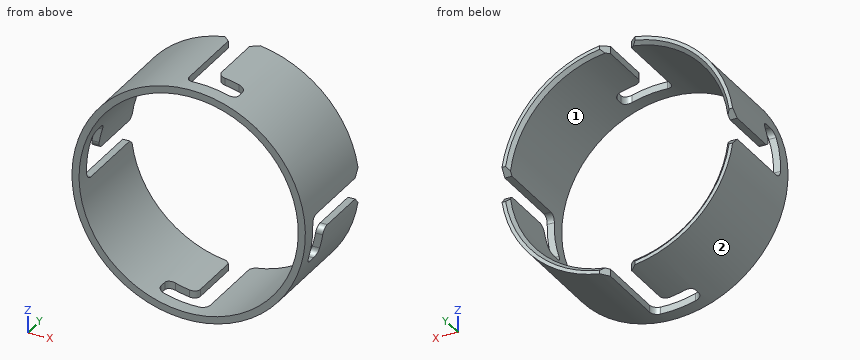
from build123d import *

# Parameters (mm, degrees)
SKETCH2_W                    = 5
SKETCH2_H                    = 72.15
CUT_EXTRUDE1_DEPTH           = 83.55
FILLET1_R                    = 5
CHAMFER1_SIZE                = 5
FILLET3_R                    = 5
CIRPATTERN1_COUNT            = 4
FILLET1_OF_CIRPATTERN1_R     = 5
CHAMFER1_OF_CIRPATTERN1_SIZE = 5
FILLET3_OF_CIRPATTERN1_R     = 5
CHAMFER2_SIZE                = 2.5


with BuildPart() as part:
    # Sketch2 → Revolve1 (revolve)
    with BuildSketch(Plane(origin=(0, 0, 0), x_dir=(0, 0, -1), z_dir=(1, 0, 0))):
        with Locations((-80.05, 36.075)):
            Rectangle(SKETCH2_W, SKETCH2_H)
    revolve(axis=Axis((0, -3.6075, 0), (0, 1, 0)))

    # Sketch3 → Cut-Extrude1 (cut, through all)
    with BuildSketch(Plane(origin=(0, 0, 0), x_dir=(0, 0, -1), z_dir=(1, 0, 0))):
        Polygon((-7.5, 72.15), (7.5, 72.15), (7.5, 10), (-27.5, 10), (-27.5, 25), (-7.5, 25), align=None)
    cut_extrude1 = extrude(amount=-CUT_EXTRUDE1_DEPTH, mode=Mode.SUBTRACT)

    # Fillet1
    fillet1_edges = [part.edges().sort_by_distance(p)[0] for p in [
        (-79.697535069, 10, -7.5),
        (-79.697535069, 25, 7.5),
    ]]
    fillet(fillet1_edges, radius=FILLET1_R)

    # Chamfer1
    chamfer1_edges = [part.edges().sort_by_distance(p)[0] for p in [
        (-79.697535069, 72.15, -7.5),
        (-79.697535069, 72.15, 7.5),
    ]]
    chamfer(chamfer1_edges, length=CHAMFER1_SIZE)

    # Fillet3
    fillet3_edges = [part.edges().sort_by_distance(p)[0] for p in [
        (-75.17256913, 10, 27.5),
        (-75.17256913, 25, 27.5),
    ]]
    fillet(fillet3_edges, radius=FILLET3_R)

    # CirPattern1: Cut-Extrude1 ×4 about axis
    cirpattern1_axis = Axis((0, 0, 0), (0, 1, 0))
    for i in range(1, CIRPATTERN1_COUNT):
        add(cut_extrude1.rotate(cirpattern1_axis, i * 360 / CIRPATTERN1_COUNT), mode=Mode.SUBTRACT)

    # Fillet1 of CirPattern1
    fillet1_of_cirpattern1_edges = [part.edges().sort_by_distance(p)[0] for p in [
        (-7.5, 10, 79.697535069),
        (7.5, 25, 79.697535069),
        (79.697535069, 10, 7.5),
        (79.697535069, 25, -7.5),
        (7.5, 10, -79.697535069),
        (-7.5, 25, -79.697535069),
    ]]
    fillet(fillet1_of_cirpattern1_edges, radius=FILLET1_OF_CIRPATTERN1_R)

    # Chamfer1 of CirPattern1
    chamfer1_of_cirpattern1_edges = [part.edges().sort_by_distance(p)[0] for p in [
        (-7.5, 72.15, 79.697535069),
        (7.5, 72.15, 79.697535069),
        (79.697535069, 72.15, 7.5),
        (79.697535069, 72.15, -7.5),
        (7.5, 72.15, -79.697535069),
        (-7.5, 72.15, -79.697535069),
    ]]
    chamfer(chamfer1_of_cirpattern1_edges, length=CHAMFER1_OF_CIRPATTERN1_SIZE)

    # Fillet3 of CirPattern1
    fillet3_of_cirpattern1_edges = [part.edges().sort_by_distance(p)[0] for p in [
        (27.5, 10, 75.17256913),
        (27.5, 25, 75.17256913),
        (75.17256913, 10, -27.5),
        (75.17256913, 25, -27.5),
        (-27.5, 10, -75.17256913),
        (-27.5, 25, -75.17256913),
    ]]
    fillet(fillet3_of_cirpattern1_edges, radius=FILLET3_OF_CIRPATTERN1_R)

    # Chamfer2
    chamfer2_edges = [part.edges().sort_by_distance(p)[0] for p in [
        (-54.836130881, 72.15, -54.836130881),
        (54.836130881, 72.15, -54.836130881),
        (54.836130881, 72.15, 54.836130881),
        (-54.836130881, 72.15, 54.836130881),
    ]]
    chamfer(chamfer2_edges, length=CHAMFER2_SIZE)


solid = part.part
The listing builds one solid part. Answer for the finished solid, in the listing's coordinates (mm). Face numbers are marked on the shaded views. Round coordinates to 2 decimals unless told otherwise and drop trailing zeros. Write each loop counter-clockwise with the first axis right and the second up, starting at its lowest first coordinate (ties: lowest second). Pieces come first, ordered by that corner, then holes. Notation, with made-up numbers: (26, 78) - (51, 78) arc R19 cw to (51, 103) - close; hole circle Ø4 at (88, 39). An arc over 180 degrees is marked (long way). Use a Markdown table: item, result. Add a question column.
1. For a pull along Z with two mould halves and no side action, classify the marked faces 1 and 2 as +Z half, -Z half, draft (parallel to the pull), parting line (faces both ways), or undercut.
2. The part is cut by section A-A (z = 0). Write down the section's boundary in (x, y), and give its area (3 significant figures).
3. Flat-ended cylindrical pins translate along their axes: P1, Ø5.5, axis at y = 43, z = 79, coming from the +X side; P2, Ø5, axis at y = 63, z = 59.5, coming from the -X side; P3, Ø4, axis at x = 40.5, y = 15.5, coming from the +Z side; P4, Ø8, axis at x = -76.5, z = 16, coming from the -Y side. Find the tip coordinate at first contact, or state that the pin passes through.
4. Consider line 1 (X direction, y = 27, z = -38.5); line 2 (X direction, y = 25.5, z = 11.5); line 3 (Z direction, x = -30, y = 34). Determine where each line is inside the solid, lowest interval first.
5. The part is cut by section D-D (z = -20.5). Give the number of separate pieces and of enclosed holes in the cut face, and give its area (3 significant figures).
6. The part is cut by section B-B (x = 0). Write down the section's boundary in (y, z), and give its area (3 significant figures).
7. The part is cut by section C-C (y = 33.5). Write down the section's boundary in (x, z), and give its area (3 significant figures).
Reported:
| question | item | result |
|---|---|---|
| 1 | face 1 | undercut |
| 1 | face 2 | parting line |
| 2 | outline | (-82.55, 0) - (-77.55, 0) - (-77.55, 10) - (-82.55, 10) - close; (77.55, 0) - (82.55, 0) - (82.55, 10) - (77.55, 10) - close |
| 2 | area | 100 mm^2 |
| 3 | P1 | x = 31.63 |
| 3 | P2 | x = -59.71 |
| 3 | P3 | z = 73.02 |
| 3 | P4 | y = 0 |
| 4 | line 1 | -73.02 to -67.32, 67.32 to 73.02 |
| 4 | line 2 | -81.75 to -76.69, 76.69 to 81.75 |
| 4 | line 3 | -76.91 to -71.51, 71.51 to 76.91 |
| 5 | separate pieces | 3 |
| 5 | enclosed holes | 0 |
| 5 | area | 662 mm^2 |
| 6 | outline | (0, -82.55) - (10, -82.55) - (10, -77.55) - (0, -77.55) - close; (0, 77.55) - (10, 77.55) - (10, 82.55) - (0, 82.55) - close |
| 6 | area | 100 mm^2 |
| 7 | outline | (-82.21, -7.5) arc R82.55 ccw to (-7.5, -82.21) - (-7.5, -77.19) arc R77.55 cw to (-77.19, -7.5) - close; (-82.21, 7.5) - (-77.19, 7.5) arc R77.55 cw to (-7.5, 77.19) - (-7.5, 82.21) arc R82.55 ccw to start; (7.5, -82.21) arc R82.55 ccw to (82.21, -7.5) - (77.19, -7.5) arc R77.55 cw to (7.5, -77.19) - close; (7.5, 77.19) arc R77.55 cw to (77.19, 7.5) - (82.21, 7.5) arc R82.55 ccw to (7.5, 82.21) - close |
| 7 | area | 2,210 mm^2 |
